from build123d import *

# Parameters (mm, degrees)
SKETCH1_W           = 9
SKETCH1_H           = 42
SKETCH1_R           = 2.02
SKETCH1_R_2         = 1.5875
BOSS_EXTRUDE1_DEPTH = 40
SKETCH1_3_R         = 2.02
SKETCH1_3_R_2       = 1.5875
CUT_EXTRUDE1_DEPTH  = 8
SKETCH2_W           = 40
SKETCH2_H           = 3
CUT_EXTRUDE2_DEPTH  = 6
CUT_EXTRUDE3_DEPTH  = 9
CUT_EXTRUDE6_DEPTH  = 7
SKETCH6_R           = 2.0193
CUT_EXTRUDE5_DEPTH  = 20
FILLET2_R           = 0.5
CHAMFER4_SIZE       = 3
SKETCH7_W           = 74.310151154
SKETCH7_H           = 95.165931092
CUT_EXTRUDE7_DEPTH  = 9
FILLET3_R           = 0.5


with BuildPart() as part:
    # Sketch1 → Boss-Extrude1 (new body)
    # profile 1 of 4: a face of its own
    with BuildSketch(Plane.XY):
        with Locations((4.5, 21)):
            Rectangle(SKETCH1_W, SKETCH1_H)
        with Locations((4.5, 16)):
            Circle(SKETCH1_R, mode=Mode.SUBTRACT)
        with Locations((4.5, 28)):
            Circle(SKETCH1_R, mode=Mode.SUBTRACT)
    # profile 2 of 4: a face of its own
    with BuildSketch(Plane.XY):
        with Locations((4.5, 28)):
            Circle(SKETCH1_R)
    # profile 3 of 4: a face of its own
    with BuildSketch(Plane.XY):
        with Locations((4.5, 16)):
            Circle(SKETCH1_R)
    # profile 4 of 4: a face of its own
    with BuildSketch(Plane.XY):
        with Locations((4.5, 35)):
            Circle(SKETCH1_R_2)
    extrude(amount=BOSS_EXTRUDE1_DEPTH)

    # Sketch1<3> → Cut-Extrude1 (cut)
    with BuildSketch(Plane.XY):
        with Locations((4.5, 28)):
            Circle(SKETCH1_3_R)
        with Locations((4.5, 35)):
            Circle(SKETCH1_3_R_2)
        with Locations((4.5, 16)):
            Circle(SKETCH1_3_R)
    extrude(amount=CUT_EXTRUDE1_DEPTH, mode=Mode.SUBTRACT)

    # Sketch2 → Cut-Extrude2 (cut)
    with BuildSketch(Plane(origin=(9, 0, 0), x_dir=(0, 0, -1), z_dir=(1, 0, 0))):
        with Locations((-20, 6.2)):
            Rectangle(SKETCH2_W, SKETCH2_H)
    extrude(amount=-CUT_EXTRUDE2_DEPTH, mode=Mode.SUBTRACT)

    # Sketch3 → Cut-Extrude3 (cut)
    with BuildSketch(Plane(origin=(9, 0, 0), x_dir=(0, 0, -1), z_dir=(1, 0, 0))):
        Polygon((-20, 42), (-40, 15), (-48.379363257, 51.913157268), align=None)
    extrude(amount=-CUT_EXTRUDE3_DEPTH, mode=Mode.SUBTRACT)

    # Sketch5 → Cut-Extrude6 (cut)
    with BuildSketch(Plane.ZY.offset(-9)):
        Polygon((20, 42), (10, 42), (10, 14.1), (40, 14.1), (40, 15), align=None)
    extrude(amount=CUT_EXTRUDE6_DEPTH, mode=Mode.SUBTRACT)

    # Sketch6 → Cut-Extrude5 (cut)
    with BuildSketch(Plane.XZ):
        with Locations(Location((6, 35, 0), (0, 0, 90))):
            Circle(SKETCH6_R)
        with Locations(Location((6, 20, 0), (0, 0, 90))):
            Circle(SKETCH6_R)
    extrude(amount=-CUT_EXTRUDE5_DEPTH, mode=Mode.SUBTRACT)

    # Fillet2
    fillet2_edges = [part.edges().sort_by_distance(p)[0] for p in [
        (0, 0, 20),
        (0, 7.5, 40),
        (0, 42, 10),
        (0, 28.5, 30),
        (0, 21, 0),
    ]]
    fillet(fillet2_edges, radius=FILLET2_R)

    # Chamfer4
    chamfer4_edges = [part.edges().sort_by_distance(p)[0] for p in [
        (9, 2.35, 40),
        (9, 10.9, 40),
    ]]
    chamfer(chamfer4_edges, length=CHAMFER4_SIZE)

    # Mirror1: part across plane


with BuildPart() as part_1:
    add(part.part)
    add(part.part.mirror(Plane(origin=(9, 0, 40), x_dir=(0, 0, 1), z_dir=(-1, 0, 0))))

    # Sketch7 → Cut-Extrude7 (cut)
    with BuildSketch(Plane.ZY):
        with Locations((29.906214843, 26.493385896)):
            Rectangle(SKETCH7_W, SKETCH7_H)
    extrude(amount=-CUT_EXTRUDE7_DEPTH, mode=Mode.SUBTRACT)

    # Fillet3
    fillet3_edges = [part_1.edges().sort_by_distance(p)[0] for p in [
        (16, 42, 15),
        (16, 14.55, 40),
        (14, 14.1, 40),
        (16, 28.5, 30),
        (16, 14.1, 25),
        (16, 28.05, 10),
        (9, 2.35, 37),
        (9, 10.9, 37),
        (12.5, 42, 10),
        (9, 2.35, 0),
        (9, 0, 18.5),
        (9, 4.7, 18.5),
        (9, 24.85, 0),
        (9, 7.7, 18.5),
        (9, 42, 5),
        (9, 28.05, 10),
        (9, 14.1, 23.5),
    ]]
    fillet(fillet3_edges, radius=FILLET3_R)


solid = part_1.part
CAD build for the part. Positions are in the model's coordinates, mm. A direction names the side the tool comes from. Round coordinates to 2 decimals unless told otherwise and drop trailing zeros. Write each loop counter-clockwise with the first axis right and the second up, starting at its lowest first coordinate (ties: lowest second). Pieces come first, ordered by that corner, then holes. Notation, with made-up numbers: M 71.5,26 L 123.5,26 A27 cw 123.5,56 Z; hole C -6,-31.75 d1. An arc over 180 degrees is marked long. Put each result on its own line as item: value. Start each with the question number.
1) Pull direction X, two halves, no side cores. Call faces 1 (the cylindrical face through (11.634, 15.226, 3.944)), 2 (the cylindrical face through (17.86, 28.22, 30.02)), 3 (the flat face through (16, 25, 22)), 4 (the cylindrical face through (11.227, 2.317, 36.865)): pulls with the +X half, pulls with the -X half, needs draft (parallel to the pull), parting line crosses it, or undercut.
2) 3-axis set-ups, long thin cutter, end or side, ignore diameter. For faces 5 (the flat face through (12, 28, 10)), 6 (the flat face through (15, 6, 20)), 7 (the flat face through (9, 2, 18)), 8 (the flat face through (14, 35, 8)): which of +Z, -Z, +X, -X, +Y, -Y reach the whole face in a straight line?
3) Saw through at B-B, the plane z = 15. Write the cut outline in (x, y), and give its area (3 significant figures).
4) Saw through at A-A, the plane z = 5.5. Write the cut outline in (x, y) (1 decimal), and give its area (3 significant figures).
5) Pin check, flat tips, straight feed: pin 1 Ø1 at (x, z) = (14.5, 18.5) entering from +Y; pin 2 Ø3 at (x, y) = (13.5, 35) entering from -Z; pin 3 Ø4 at (x, y) = (10.5, 27) entering from +Z. Stop position of each tip, or through.
6) Drill centre lines: probe 1 along Y at (x, z) = (10.75, 5); probe 2 along Y at (x, z) = (10.25, 31.5); probe 3 along Y at (x, z) = (13.5, 2). Where is each one in solid material? Low to high. Write a range as [from, to].
7) Saw through at D-D, the plane x = 10.5. Write the cut outline in (y, z).
8) Saw through at C-C, the plane y = 10.5. Write the cut outline in (x, z), and give its area (3 significant figures).
Resolved:
1. face 1: undercut
1. face 2: pulls with the +X half
1. face 3: pulls with the -X half
1. face 4: undercut
2. face 5: +Z, -X, +Y
2. face 6: +Z, -Z, -X
2. face 7: +Z, -Z, -X, +Y, -Y
2. face 8: -Z
3. outline: M 9,0.5 A0.5 ccw 9.5,0 L 17.5,0 A0.5 ccw 18,0.5 L 18,41.5 A0.5 ccw 17.5,42 L 16.5,42 A0.5 ccw 16,41.5 L 16,14.6 A0.5 cw 15.5,14.1 L 9.5,14.1 A0.5 ccw 9,13.6 L 9,8.2 A0.5 ccw 9.5,7.7 L 15,7.7 L 15,4.7 L 9.5,4.7 A0.5 ccw 9,4.2 Z
3. area: 164 mm²
4. outline: M 9,0.5 A0.5 ccw 9.5,0 L 17.5,0 A0.5 ccw 18,0.5 L 18,41.5 A0.5 ccw 17.5,42 L 9.5,42 A0.5 ccw 9,41.5 L 9,8.2 A0.5 ccw 9.5,7.7 L 15,7.7 L 15,4.7 L 9.5,4.7 A0.5 ccw 9,4.2 Z; hole C 13.5,16 d4; hole C 13.5,28 d4; hole C 13.5,35 d3.2
4. area: 326 mm²
5. pin 1: y = 14.1
5. pin 2: z = 8
5. pin 3: z = 10
6. probe 1: [0, 4.7], [7.7, 42]
6. probe 2: [0, 4.7], [7.7, 14.1]
6. probe 3: [0, 4.7], [7.7, 13.98], [18.02, 25.98], [30.02, 33.41], [36.59, 42]
7. outline: M 0,0 L 4.7,0 L 4.7,18.65 L 0,18.65 Z; M 0,21.35 L 4.7,21.35 L 4.7,33.65 L 0,33.65 Z; M 0,36.35 L 4.7,36.35 L 4.7,38.5 L 0,38.5 Z; M 7.7,0 L 42,0 L 42,9.5 A0.5 ccw 41.5,10 L 14.1,10 L 14.1,18.65 L 7.7,18.65 Z; M 7.7,21.35 L 14.1,21.35 L 14.1,33.65 L 7.7,33.65 Z; M 7.7,36.35 L 14.1,36.35 L 14.1,38.5 L 7.7,38.5 Z
8. outline: M 9,0.5 A0.5 ccw 9.5,0 L 17.5,0 A0.5 ccw 18,0.5 L 18,39.5 A0.5 ccw 17.5,40 L 12,40 L 9.15,37.15 A0.5 ccw 9,36.79 Z; hole C 12,20 d4.04; hole C 12,35 d4.04
8. area: 330 mm²
